```python
from build123d import *

# Parameters (mm, degrees)
F0_W     = 75
F0_H     = 75
F0_W_2   = 50
F0_H_2   = 50
F1_DEPTH = 2
F2_DEPTH = 3
F3_W     = 1
F3_H     = 5
F3_W_2   = 5
F3_H_2   = 1
F3_W_3   = 63
F3_H_3   = 63
F4_DEPTH = 1


with BuildPart() as f1:
    # F0 (on Top) → F1 (new body)
    with BuildSketch(Plane.XY):
        Rectangle(F0_W, F0_H)
        Rectangle(F0_W_2, F0_H_2, mode=Mode.SUBTRACT)
        Rectangle(F0_W_2, F0_H_2)
    extrude(amount=F1_DEPTH)

    # F0 (on Top) → F2 (join)
    with BuildSketch(Plane.XY):
        Rectangle(F0_W_2, F0_H_2)
    extrude(amount=F2_DEPTH)

    # F3 (on face) → F4 (cut)
    with BuildSketch(Plane.XY):
        with Locations((-32, -35)):
            Rectangle(F3_W, F3_H)
        with Locations((-35, -32)):
            Rectangle(F3_W_2, F3_H_2)
        with Locations((-32, -32)):
            Rectangle(F3_W, F3_H_2)
        with Locations((0, -32)):
            Rectangle(F3_W_3, F3_H_2)
        with Locations((-32, 0)):
            Rectangle(F3_W, F3_H_3)
        with Locations((32, -32)):
            Rectangle(F3_W, F3_H_2)
        with Locations((32, -35)):
            Rectangle(F3_W, F3_H)
        with Locations((-35, 32)):
            Rectangle(F3_W_2, F3_H_2)
        with Locations((-32, 32)):
            Rectangle(F3_W, F3_H_2)
        with Locations((0, 32)):
            Rectangle(F3_W_3, F3_H_2)
        with Locations((32, 0)):
            Rectangle(F3_W, F3_H_3)
        with Locations((35, -32)):
            Rectangle(F3_W_2, F3_H_2)
        with Locations((-32, 35)):
            Rectangle(F3_W, F3_H)
        with Locations((32, 32)):
            Rectangle(F3_W, F3_H_2)
        with Locations((32, 35)):
            Rectangle(F3_W, F3_H)
        with Locations((35, 32)):
            Rectangle(F3_W_2, F3_H_2)
    extrude(amount=F4_DEPTH, mode=Mode.SUBTRACT)


solid = f1.part
```
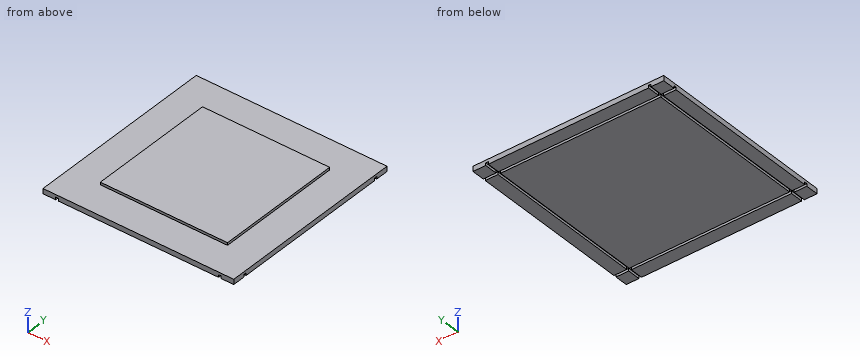
The model under review builds one solid part; all positions refer to its coordinate system, in mm. Round coordinates to 2 decimals unless told otherwise and drop trailing zeros. Order: outer loops, then holes, each group sorted by start corner. A loop starts at its lowest first (then second) coordinate and runs counter-clockwise, first axis right, second up. Notation, with made-up numbers: (-21, 27.25) -> (6, 27.25) arc R22 ccw to (6, 64.25) -> close; hole circle Ø4 at (79.25, 33). An arc over 180 degrees is marked (long way). One line per item, written item: value. Start each with the question number.
Q1. Take a section at A-A (x = -29). Write out the cut boundary in (y, z).
Q2. Take a section at B-B (y = -1.5). Write out the cut boundary in (x, z), and give its area (3 significant figures).
Q3. Clearance check with a flat-ended pin moving along its axis: pin 1 Ø1 at (x, y) = (-17.5, 26) entering from +Z. State where the tip first meets the part, or that it passes through.
Q4. Wall thickness on line 1 (X direction, y = -14, z = 0.65); line 2 (Z direction, x = -22.5, y = 31): over which ranges is each line inside the solid? List them lowest first.
Q5. Take a section at C-C (z = 2.5). Write out the cut boundary in (x, y), and give its area (3 significant figures).
Reported:
1. outline: (-37.5, 0) -> (-32.5, 0) -> (-32.5, 1) -> (-31.5, 1) -> (-31.5, 0) -> (31.5, 0) -> (31.5, 1) -> (32.5, 1) -> (32.5, 0) -> (37.5, 0) -> (37.5, 2) -> (-37.5, 2) -> close
2. outline: (-37.5, 0) -> (-32.5, 0) -> (-32.5, 1) -> (-31.5, 1) -> (-31.5, 0) -> (31.5, 0) -> (31.5, 1) -> (32.5, 1) -> (32.5, 0) -> (37.5, 0) -> (37.5, 2) -> (25, 2) -> (25, 3) -> (-25, 3) -> (-25, 2) -> (-37.5, 2) -> close
2. area: 198 mm2
3. pin 1: stops at z = 2
4. line 1: x = -37.5 to -32.5, -31.5 to 31.5, 32.5 to 37.5
4. line 2: z = 0 to 2
5. outline: (-25, -25) -> (25, -25) -> (25, 25) -> (-25, 25) -> close
5. area: 2,500 mm2
